The listing builds one solid part. Answer for the finished solid, in the listing's coordinates (mm). Face numbers are marked on the shaded views. A direction names the side the tool comes from. Give positions to 0.01 mm unless a question says otherwise; leave off trailing zeros. Loops run counter-clockwise (first coordinate to the right, second up) from the corner with the lowest first, then second, coordinate; pieces in that order, holes last. Notation, with made-up numbers: (5, 5) - (49, 5) arc R15 ccw to (49, 27) - close; hole circle Ø5 at (71.5, 16.25). An arc over 180 degrees is marked (long way). Write each question's results on one line, items separated by ' | '.
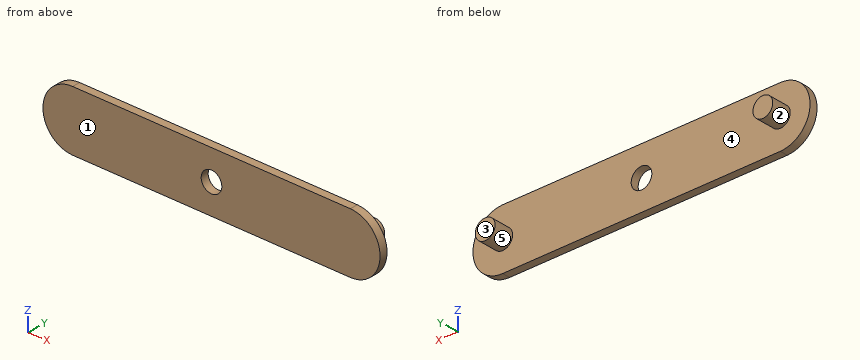
from build123d import *

# Parameters (mm, degrees)
SKETCH1_W           = 88.9
SKETCH1_H           = 19.05
BOSS_EXTRUDE1_DEPTH = 2.54
SKETCH2_R           = 3.175
BOSS_EXTRUDE2_DEPTH = 6.35
CUT_EXTRUDE1_REACH  = 57.176
SKETCH3_R           = 3.302


with BuildPart() as part:
    # Sketch1 → Boss-Extrude1 (new body)
    with BuildSketch(Plane(origin=(0, 0, 0), x_dir=(1, 0, 0), z_dir=(0, 1, 0))):
        with BuildLine():
            ThreePointArc((-44.45, -9.525), (-53.975, 0), (-44.45, 9.525))
            Line((-44.45, 9.525), (-44.45, -9.525))
        make_face()
        Rectangle(SKETCH1_W, SKETCH1_H)
        with BuildLine():
            ThreePointArc((44.45, 9.525), (53.975, 0), (44.45, -9.525))
            Line((44.45, -9.525), (44.45, 9.525))
        make_face()
    extrude(amount=BOSS_EXTRUDE1_DEPTH)

    # Sketch2 → Boss-Extrude2 (add)
    with BuildSketch(Plane(origin=(0, 2.54, 0), x_dir=(1, 0, 0), z_dir=(0, 1, 0))):
        with Locations(Location((-44.45, 0, 0), (0, 0, 270))):
            Circle(SKETCH2_R)
        with Locations(Location((44.45, 0, 0), (0, 0, 270))):
            Circle(SKETCH2_R)
    extrude(amount=BOSS_EXTRUDE2_DEPTH)

    # Sketch3 → Cut-Extrude1 (cut, up to next)
    with BuildSketch(Plane(origin=(0, 2.54, 0), x_dir=(1, 0, 0), z_dir=(0, 1, 0)), mode=Mode.PRIVATE) as cut_extrude1_sk1:
        with Locations(Location((0, 0, 0), (0, 0, 270))):
            Circle(SKETCH3_R)
    cut_extrude1_tool1 = extrude(cut_extrude1_sk1.sketch, amount=-CUT_EXTRUDE1_REACH, mode=Mode.PRIVATE) & part.part
    add(cut_extrude1_tool1.solids().sort_by_distance((0, 2.54, 0))[0], mode=Mode.SUBTRACT)


solid = part.part
Item 1: Find the intervals of material crossed by line 1 along X through (y, z) = (1.05, 0) (3 decimals); line 2 along Y through (x, z) = (-4, 3.5); line 3 along Z through (x, y) = (45, 2.5), in increasing order. Write a range as [from, to].
Values found:
line 1: x = [-53.975, -3.302], [3.302, 53.975] | line 2: y = [0, 2.54] | line 3: z = [-9.51, 9.51]
Item 2: A cutting plane is placed at B-B, the plane z = 0. Determine the outline of the cut face in (x, y) (3 decimals), plus the area to 3 significant figures.
Values found:
outline: (-53.975, 0) - (-3.302, 0) - (-3.302, 2.54) - (-41.275, 2.54) - (-41.275, 8.89) - (-47.625, 8.89) - (-47.625, 2.54) - (-53.975, 2.54) - close; (3.302, 0) - (53.975, 0) - (53.975, 2.54) - (47.625, 2.54) - (47.625, 8.89) - (41.275, 8.89) - (41.275, 2.54) - (3.302, 2.54) - close | area: 338 mm²
Item 3: For the marked faces 1 and 2, determine the directions among +Z, -Z, +X, -X, +Y, -Y from which every point of the face is accessible in a straight line to the end or side of a thin tool.
Values found:
face 1: +Z, -Z, +X, -X, -Y | face 2: +Y
Item 4: Flat-ended cylindrical pins translate along their axes: P1, Ø4, axis at x = -26, z = 2.5, coming from the +Y side; P2, Ø4, axis at y = 3, z = 4, coming from the -X side; P3, Ø2, axis at y = 5, z = -0.5, coming from the +X side (3 decimals). Find the tip coordinate at first contact, or state that the pin passes through.
Values found:
P1: stops at y = 2.54 | P2: stops at x = -53.75 | P3: stops at x = 47.625
Item 5: For a pull along X with two mould halves and no side action, classify the marked faces 3, 4 and 5 as released by +X, released by -X, zero draft, split by the parting line, or undercut.
Values found:
face 3: zero draft | face 4: undercut | face 5: undercut
Item 6: A cutting plane is placed at C-C, the plane y = 1.5. Determine the outline of the cut face in (x, z) (3 decimals), plus the area to 3 significant figures.
Values found:
outline: (-44.45, -9.525) - (44.45, -9.525) arc R9.525 ccw to (44.45, 9.525) - (-44.45, 9.525) arc R9.525 ccw to start; hole circle Ø6.604 at (0, 0) | area: 1,940 mm²
Item 7: A cutting plane is placed at A-A, the plane x = 0. Determine the outline of the cut face in (y, z) (3 decimals), plus the area to 3 significant figures.
Values found:
outline: (0, -9.525) - (2.54, -9.525) - (2.54, -3.302) - (0, -3.302) - close; (0, 3.302) - (2.54, 3.302) - (2.54, 9.525) - (0, 9.525) - close | area: 31.6 mm²
Item 8: A cutting plane is placed at D-D, the plane y = 6.25. Determine the outline of the cut face in (x, z) (3 decimals).
Values found:
outline: circle Ø6.35 at (-44.45, 0); circle Ø6.35 at (44.45, 0)
